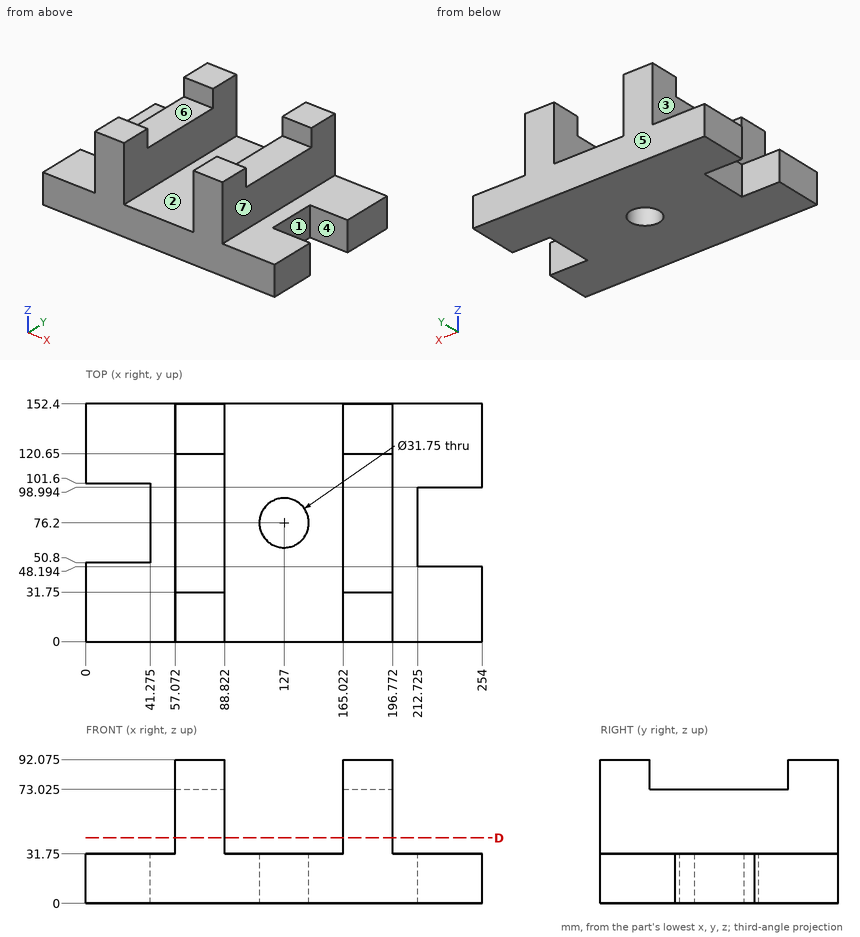
The drawing under review shows one solid part. Ordinate dimensions are in mm from its lowest x, y, z. A direction names the side the tool comes from. Give positions to 0.01 mm unless a question says otherwise; leave off trailing zeros. Loops run counter-clockwise (first coordinate to the right, second up) from the corner with the lowest first, then second, coordinate; pieces in that order, holes last. Notation, with made-up numbers: M 84,85 L 99,85 A21 cw 99,116 Z; hole C 78.5,-17.5 d8. An arc over 180 degrees is marked long. One line per item, written item: value. Start each with the question number.
Q1. Machinability: for the marked faces 1, 2 and 3, which of the approach directions +Z, -Z, +X, -X, +Y, -Y give a long, thin tool a straight path to every point of the face, cutting with its end or side? Answer none if there is none.
Q2. Draft analysis for pull direction Y (two halves, no side actions). For the marked faces 4, 5, 6 and 7, state which applies: released by +Y, released by -Y, zero draft, split by the parting line, or undercut.
Q3. Clearance check with flat-ended pins moving along their axes: pin 1 Ø10 at (y, z) = (111, 62.5) entering from +X; pin 2 Ø6 at (x, y) = (166.5, 57.5) entering from +Z (3 decimals); pin 3 Ø3 at (x, y) = (110.5, 132) entering from +Z. State where each tip first meets the part, or that it passes through.
Q4. For L1, parallel to Y at x = 214, z = 19 (1 decimal); L2, parallel to Y at x = 127, z = 7 (1 decimal); L3, parallel to X at y = 122, z = 60, list the stretches that pass through material, from the lowest coordinate up.
Q5. Add section D-D (z = 42). Give the boundary of the cut face in (x, y).
Reply:
1. face 1: +Z, -Z, +X
1. face 2: +Z, +Y, -Y
1. face 3: +Z, -X, +Y, -Y
2. face 4: undercut
2. face 5: released by +Y
2. face 6: undercut
2. face 7: zero draft
3. pin 1: x = 196.77
3. pin 2: z = 73.025
3. pin 3: z = 31.75
4. L1: 0 to 48.2, 99 to 152.4
4. L2: 0 to 60.3, 92.1 to 152.4
4. L3: 57.07 to 88.82, 165.02 to 196.77
5. outline: M 57.07,0 L 88.82,0 L 88.82,152.4 L 57.07,152.4 Z; M 165.02,0 L 196.77,0 L 196.77,152.4 L 165.02,152.4 Z
